Could you check a few things on this model? Use its own coordinates, in mm. A direction names the side the tool comes from. Give positions to 0.01 mm unless a question says otherwise; leave off trailing zeros. Loops run counter-clockwise (first coordinate to the right, second up) from the corner with the lowest first, then second, coordinate; pieces in that order, holes last. Notation, with made-up numbers: (83, 84.5) - (106, 84.5) arc R21 ccw to (106, 115.5) - close; hole circle Ø1 at (-34.5, 77). An arc over 180 degrees is marked (long way). One line per item, written item: value. Start each with the question number.
Q1. For faces 4 (the face through (-2, 2, -1)), 5 (the face through (0, 2, -4.5)), 6 (the face through (2, 2, -5)), 7 (the face through (0, 2, 1)), which set-ups out of +Z, -Z, +X, -X, +Y, -Y let a thin tool reach every point of the face, with its end or its side?
Q2. I'm going to push flat-ended pins straight in: P1, Ø0.8, axis at x = -8.5, y = 1.5, coming from the -Z side; P2, Ø0.8, axis at y = 2, z = 3, coming from the -X side; P3, Ø6, axis at x = -8, z = -2.5, coming from the +Y side; P4, Ø2.5, axis at x = -7.5, z = -5.5, coming from the +Y side. Where does each tip first touch, or does it pass through?
Q3. I want a section at A-A (y = 1.55). Please give me the cut outline in (x, z), then the cut area to 3 significant figures.
Q4. I want a section at D-D (y = 0.4). Please give me the cut outline in (x, z), then the cut area to 3 significant figures.
Q5. If I drill on line 1 (X direction, y = 0.6, z = -5.5); line 2 (Y direction, x = -2.5, z = -3); line 3 (Z direction, x = 8.75, y = 0.7), over which ranges is the centre line in solid material (lowest first)? Write a range as from..to.
Q6. I want a section at C-C (z = -5.5). Please give me the cut outline in (x, y).
Q7. I want a section at B-B (x = 7.5). Please give me the cut outline in (y, z).
Q8. If we mould it in two halves opening along X, with no side actions, what happens to faces 1 (the face through (6.036, 0.493, -5.825)), 2 (the face through (-8, 2, 2.2)), 3 (the face through (-9.5, 2, 3))? For each: released by +X, released by -X, zero draft, split by the parting line, or undercut.
```python
from build123d import *

# Parameters (mm, degrees)
SKETCH1_W        = 21
SKETCH1_H        = 16
SKETCH1_R        = 1.5
PCB_DEPTH        = 1
SKETCH2_W        = 4
SKETCH2_H        = 4
SKETCH2_W_2      = 3
SKETCH2_H_2      = 1.8
COMPONENTS_DEPTH = 1.5
SKETCH3_W        = 4
SKETCH3_H        = 2
CAPACITOR_DEPTH  = 1.5


with BuildPart() as part:
    # Sketch1 → PCB (new body)
    with BuildSketch(Plane(origin=(0, 0, 0), x_dir=(1, 0, 0), z_dir=(0, 1, 0))):
        Rectangle(SKETCH1_W, SKETCH1_H)
        with Locations(Location((-7.5, 5.5, 0), (0, 0, 270))):
            Circle(SKETCH1_R, mode=Mode.SUBTRACT)
        with Locations(Location((7.5, 5.5, 0), (0, 0, 270))):
            Circle(SKETCH1_R, mode=Mode.SUBTRACT)
    extrude(amount=PCB_DEPTH)

    # Sketch2 → Components (add)
    with BuildSketch(Plane(origin=(0, 1, 0), x_dir=(1, 0, 0), z_dir=(0, 1, 0))):
        with Locations((0, 1)):
            Rectangle(SKETCH2_W, SKETCH2_H)
        with Locations((-8, -3.1)):
            Rectangle(SKETCH2_W_2, SKETCH2_H_2)
    extrude(amount=COMPONENTS_DEPTH)

    # Sketch3 → Capacitor (add)
    with BuildSketch(Plane(origin=(0, 1, 0), x_dir=(1, 0, 0), z_dir=(0, 1, 0))):
        with Locations((0, 5.5)):
            Rectangle(SKETCH3_W, SKETCH3_H)
    extrude(amount=CAPACITOR_DEPTH)


solid = part.part
```
Worked answers:
1. face 4: +Z, -Z, -X, +Y
1. face 5: +X, -X, +Y
1. face 6: +Z, -Z, +X, +Y
1. face 7: +Z, +X, -X, +Y
2. P1: stops at z = 2.2
2. P2: stops at x = -9.5
2. P3: stops at y = 1
2. P4: passes through
3. outline: (-9.5, 2.2) - (-6.5, 2.2) - (-6.5, 4) - (-9.5, 4) - close; (-2, -6.5) - (2, -6.5) - (2, -4.5) - (-2, -4.5) - close; (-2, -3) - (2, -3) - (2, 1) - (-2, 1) - close
3. area: 29.4 mm²
4. outline: (-10.5, -8) - (10.5, -8) - (10.5, 8) - (-10.5, 8) - close; hole circle Ø3 at (-7.5, -5.5); hole circle Ø3 at (7.5, -5.5)
4. area: 322 mm²
5. line 1: x = -10.5..-9, -6..6, 9..10.5
5. line 2: y = 0..1
5. line 3: z = -8..-6.33, -4.67..8
6. outline: (-10.5, 0) - (-9, 0) - (-9, 1) - (-10.5, 1) - close; (-6, 0) - (6, 0) - (6, 1) - (2, 1) - (2, 2.5) - (-2, 2.5) - (-2, 1) - (-6, 1) - close; (9, 0) - (10.5, 0) - (10.5, 1) - (9, 1) - close
7. outline: (0, -8) - (1, -8) - (1, -7) - (0, -7) - close; (0, -4) - (1, -4) - (1, 8) - (0, 8) - close
8. face 1: undercut
8. face 2: zero draft
8. face 3: released by -X
